Autodesk Inventor part; units mm, degrees
ref_plane "Work Plane1" through (0, 0, 19.05) normal (0, 0, 1) x (1, 0, 0)
ref_plane "Work Plane3" through (-11.1125, 0, 0) normal (1, 0, 0) x (0, 1, 0)
ref_plane "Work Plane5" through (-3.7562, 28.0591, 0) normal (0, 1, 0) x (-1, 0, 0)
sketch "Sketch1" plane through (0, 0, 0) normal (0, 0, 1) x (1, 0, 0)
  arc A0 (21.6438, 2.6591) -> (-3.7562, 28.0591) centre (-3.7562, 2.6591) ccw
  line L0 (-3.7562, 28.0591) -> (-3.7562, 2.6591)
  line L1 (-3.7562, 2.6591) -> (22.0131, 2.6591)
  dimension "d0" = 50.8
revolve "Revolution1" add sketch "Sketch1" angle 360 about axis through (-3.7562, 28.0591, 0) along (0, -1, 0)
ref_plane "Work Plane1" through (0, 0, 19.05) normal (0, 0, 1) x (1, 0, 0)
sketch "Sketch3" plane through (0, 0, 0) normal (0, 0, 1) x (1, 0, 0)
  line L0 (-3.675, 51.7812) -> (-3.675, -20.9618)
shell "Shell2" thickness 1.27 removed faces 1 at (1.2995, 2.6591, -4.9417)
ref_plane "Work Plane3" through (-11.1125, 0, 0) normal (1, 0, 0) x (0, 1, 0)
ref_plane "Work Plane5" through (-3.7562, 28.0591, 0) normal (0, 1, 0) x (-1, 0, 0)
sketch "Sketch12" plane through (-3.7562, 28.0591, 0) normal (0, 1, 0) x (-1, 0, 0)
  circle A0 centre (0, 0) radius 14.605
  dimension "d36" = 29.21
extrude "Extrusion8" cut sketch "Sketch12" against normal blind 25.4
properties part number "SentiBot top"
Here's how the part is built. I have some questions about the finished solid (model axes, mm). Coordinates: 2 decimals unless noted, no trailing zeros. Loops run counter-clockwise (first coordinate to the right, second up) from the corner with the lowest first, then second, coordinate; pieces in that order, holes last. Notation, with made-up numbers: (-19.75, -37.75) - (36.25, -37.75) arc R18 ccw to (36.25, -29.75) - close; hole circle Ø2 at (31, 43.5). An arc over 180 degrees is marked (long way). Return JSON: item names as keys, results as strings. Group by question number.
Item 1: If we section it at B-B on z = 0: Write out the boundary of the cut face in (x, y).
Item 2: If we section it at A-A on x = 1.5: Write out the boundary of the cut face in (y, z), and give its area (3 significant figures).
Item 3: I need wall thicknesses on line 1 (X direction, y = 14.25, z = 0.5); line 2 (X direction, y = 11.75, z = 19); line 3 (Z direction, x = -12.5, y = 19). Which ranges of each line are inside material? Lowest first, please. Write a range as from..to.
Item 4: Will these pins go through, and if not, where does the flat tip stop? P1, Ø3, axis at x = -18.5, y = 8.5, coming from the +Z side; P2, Ø10, axis at y = 6, z = -9, coming from the -X side; P3, Ø4, axis at x = -14, z = -19.5, coming from the +Y side; P4, Ø23.5, axis at x = -3.76, z = 0, coming from the -Y side.
Item 5: If we section it at D-D on z = -22: Write out the boundary of the cut face in (x, y), and give its area (3 significant figures).
Item 6: We'd pull the mould along Z, two halves only. Please class faces 1 (the face through (-1.85, 22.66, 14.48)), 2 (the face through (19, 2.659, -9)): +Z half, -Z half, draft (parallel to the pull), parting line (faces both ways), or undercut.
Item 7: If we section it at C-C on y = 10.5: Write out the boundary of the cut face in (x, z).
Calculated:
{
 "1": {"outline": "(-29.16, 2.66) - (-27.89, 2.66) arc R24.13 cw to (-18.36, 21.87) - (-18.36, 23.44) arc R25.4 ccw to start; (10.85, 21.87) arc R24.13 cw to (20.37, 2.66) - (21.64, 2.66) arc R25.4 ccw to (10.85, 23.44) - close"},
 "2": {"outline": "(2.66, -24.85) arc R24.85 ccw to (23.44, -13.63) - (21.87, -13.63) arc R23.55 cw to (2.66, -23.55) - close; (2.66, 23.55) arc R23.55 cw to (21.87, 13.63) - (23.44, 13.63) arc R24.85 ccw to (2.66, 24.85) - close", "area": "61.2 mm^2"},
 "3": {"line 1": "x = -26.35..-24.91, 17.4..18.84", "line 2": "x = -17.95..-15.53, 8.02..10.44", "line 3": "z = -17.37..-15.45, 15.45..17.37"},
 "4": {"P1": "stops at z = 20.95", "P2": "stops at x = -28.74", "P3": "stops at y = 18.28", "P4": "passes through"},
 "5": {"outline": "(-16.45, 2.66) - (-13.67, 2.66) arc R9.91 cw to (6.16, 2.66) - (8.94, 2.66) arc R12.69 ccw to start", "area": "98.8 mm^2"},
 "6": {"face 1": "undercut", "face 2": "draft"},
 "7": {"outline": "circle Ø48.32 at (-3.76, 0); hole circle Ø45.64 at (-3.76, 0)"}
}
